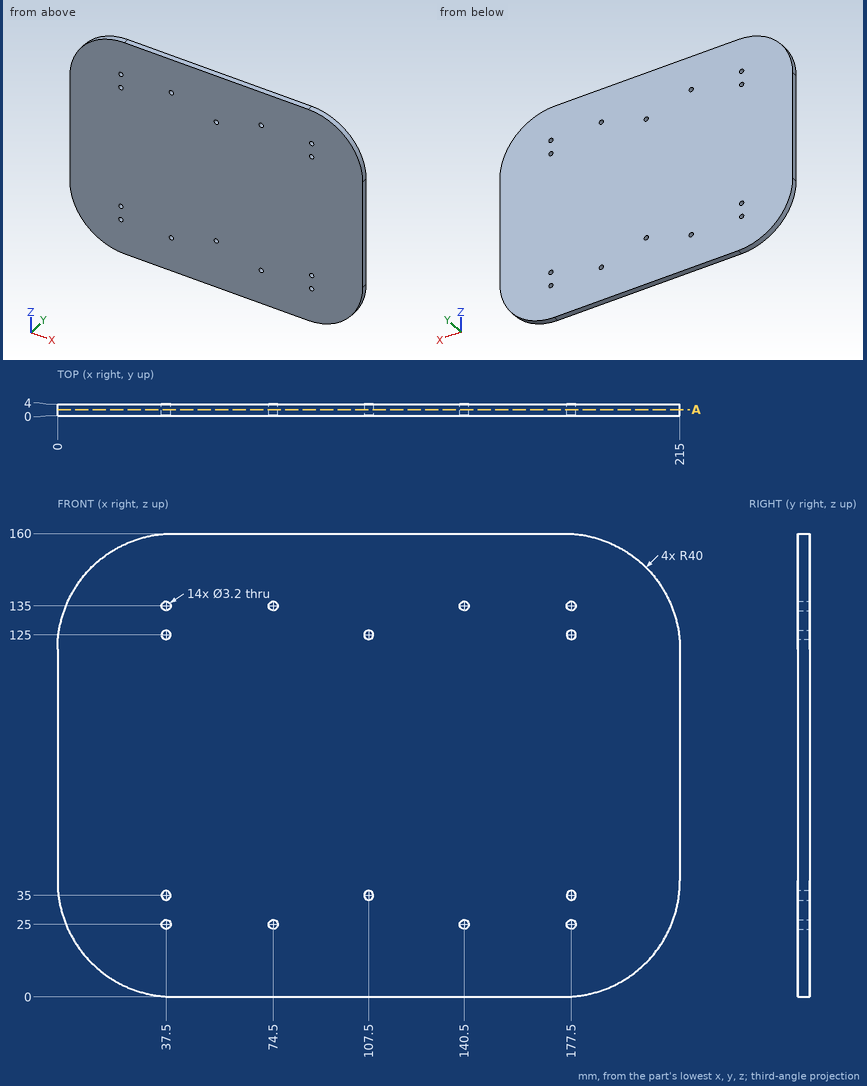
Here's the drawing with two shaded views (mm, measured from the low corner). I have some questions. Give positions to 0.01 mm unless a question says otherwise; leave off trailing zeros. One line per item, written item: value.
Q1. Suppose I cut it at A-A on y = 2.05. State how many separate pieces and enclosed holes the cut face has, then the cut area to 3 significant figures.
Answers follow:
separate pieces: 1
enclosed holes: 14
area: 32,900 mm^2
Q2. If I drill on line 1 along Z through (x, y) = (74.5, 2.5); line 2 along Z through (x, y) = (107.5, 1); line 3 along X through (y, z) = (2.5, 126), over which ranges is the centre line in solid material (lowest first)?
Answers follow:
line 1: 0 to 23.4, 26.6 to 133.4, 136.6 to 160
line 2: 0 to 33.4, 36.6 to 123.4, 126.6 to 160
line 3: 0.45 to 36.25, 38.75 to 106.25, 108.75 to 176.25, 178.75 to 214.55
Q3. I'm going to push a flat-ended pin straight in: pin 1 Ø2 at (x, y) = (30.5, 1) entering from -Z. Where does the tip first touch, or does it pass through?
Answers follow:
pin 1: z = 0.91
